```python
from build123d import *

# Parameters (mm, degrees)
SKETCH1_R           = 2.1
BOSS_EXTRUDE1_DEPTH = 360
FILLET1_R           = 0.1


with BuildPart() as part:
    # Sketch1 → Boss-Extrude1 (new body)
    with BuildSketch(Plane.XY):
        with BuildLine():
            Line((10, -19), (10, -13))
            Line((10, -13), (8, -13))
            Line((8, -13), (8, -16))
            Line((8, -16), (7, -16))
            Line((7, -16), (4, -13))
            Line((4, -13), (4, -7))
            Line((4, -7), (7, -4))
            Line((7, -4), (8, -4))
            Line((8, -4), (8, -7))
            Line((8, -7), (10, -7))
            Line((10, -7), (10, 7))
            Line((10, 7), (8, 7))
            Line((8, 7), (8, 4))
            Line((8, 4), (7, 4))
            Line((7, 4), (4, 7))
            Line((4, 7), (4, 13))
            Line((4, 13), (7, 16))
            Line((7, 16), (8, 16))
            Line((8, 16), (8, 13))
            Line((8, 13), (10, 13))
            Line((10, 13), (10, 19))
            ThreePointArc((10, 19), (9.707106781, 19.707106781), (9, 20))
            Line((9, 20), (3, 20))
            Line((3, 20), (3, 18))
            Line((3, 18), (6, 18))
            Line((6, 18), (6, 17))
            Line((6, 17), (3, 14))
            Line((3, 14), (-3, 14))
            Line((-3, 14), (-6, 17))
            Line((-6, 17), (-6, 18))
            Line((-6, 18), (-3, 18))
            Line((-3, 18), (-3, 20))
            Line((-3, 20), (-9, 20))
            ThreePointArc((-9, 20), (-9.707106781, 19.707106781), (-10, 19))
            Line((-10, 19), (-10, 13))
            Line((-10, 13), (-8, 13))
            Line((-8, 13), (-8, 16))
            Line((-8, 16), (-7, 16))
            Line((-7, 16), (-4, 13))
            Line((-4, 13), (-4, 7))
            Line((-4, 7), (-7, 4))
            Line((-7, 4), (-8, 4))
            Line((-8, 4), (-8, 7))
            Line((-8, 7), (-10, 7))
            Line((-10, 7), (-10, -7))
            Line((-10, -7), (-8, -7))
            Line((-8, -7), (-8, -4))
            Line((-8, -4), (-7, -4))
            Line((-7, -4), (-4, -7))
            Line((-4, -7), (-4, -13))
            Line((-4, -13), (-7, -16))
            Line((-7, -16), (-8, -16))
            Line((-8, -16), (-8, -13))
            Line((-8, -13), (-10, -13))
            Line((-10, -13), (-10, -19))
            ThreePointArc((-10, -19), (-9.707106781, -19.707106781), (-9, -20))
            Line((-9, -20), (-3, -20))
            Line((-3, -20), (-3, -18))
            Line((-3, -18), (-6, -18))
            Line((-6, -18), (-6, -17))
            Line((-6, -17), (-3, -14))
            Line((-3, -14), (3, -14))
            Line((3, -14), (6, -17))
            Line((6, -17), (6, -18))
            Line((6, -18), (3, -18))
            Line((3, -18), (3, -20))
            Line((3, -20), (9, -20))
            ThreePointArc((9, -20), (9.707106781, -19.707106781), (10, -19))
        make_face()
        with Locations((0, -10)):
            Circle(SKETCH1_R, mode=Mode.SUBTRACT)
        with Locations((0, 10)):
            Circle(SKETCH1_R, mode=Mode.SUBTRACT)
        Polygon((-7, -2), (-8, -2), (-8, 2), (-7, 2), (-3, 6), (3, 6), (7, 2), (8, 2), (8, -2), (7, -2), (3, -6), (-3, -6), align=None, mode=Mode.SUBTRACT)
    extrude(amount=-BOSS_EXTRUDE1_DEPTH)

    # Fillet1
    fillet1_edges = [part.edges().sort_by_distance(p)[0] for p in [
        (-10, -13, -180),
        (-10, -7, -180),
        (-10, 7, -180),
        (-10, 13, -180),
        (10, 13, -180),
        (10, 7, -180),
        (10, -7, -180),
        (10, -13, -180),
    ]]
    fillet(fillet1_edges, radius=FILLET1_R)


solid = part.part
```
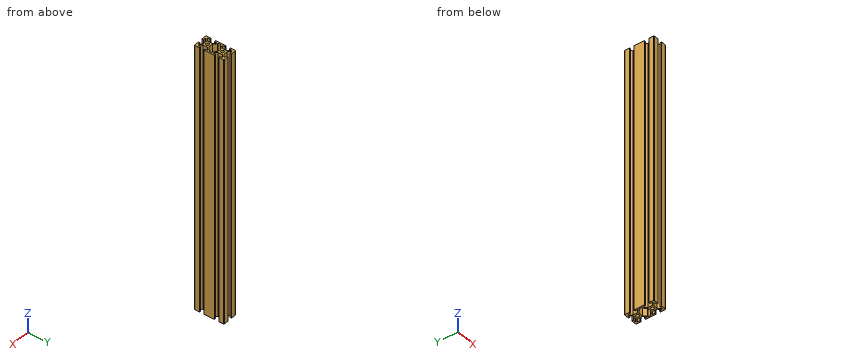
Geometry: final body of the model. Coordinates: model frame, mm. Round coordinates to 2 decimals unless told otherwise and drop trailing zeros. Use one line per item in the form item = value. Start each with the question number.
Q1. Cut plane A-A (z = -106). Count the separate pieces of the cut face and the enclosed holes in it, and give its area (3 significant figures).
Q2. Pin query (flat end, axial travel): pin 1 Ø12 at (x, y) = (-1, -3) entering from -Z; pin 2 Ø1.8 at (y, z) = (-10.5, -259.5) entering from -X. Return the tip coordinate at first contact, or that it passes through.
Q3. Material intervals for line 1 (Y direction, x = 7, z = -324); line 2 (Y direction, x = 0, z = -166); line 3 (X direction, y = 17.5, z = -190), sorted ascending. Write a range as [from, to].
Geometry results:
q1.separate_pieces = 1
q1.enclosed_holes = 3
q1.area = 321 mm^2
q2.pin_1 = -360
q2.pin_2 = -4
q3.line_1 = [-20, -16], [-4, -2], [2, 4], [16, 20]
q3.line_2 = [-14, -12.1], [-7.9, -6], [6, 7.9], [12.1, 14]
q3.line_3 = [-10, -6], [6, 10]
